```python
from build123d import *

# Parameters (mm, degrees)
SKETCH_1_W          = 20
SKETCH_1_H          = 20
EXTRUDE_1_DEPTH     = 30
SKETCH_2_R          = 5
EXTRUDE_2_DEPTH     = 50
EXTRUDE_3_DEPTH     = 20
CUT_EXTRUDE_1_REACH = 88.602
SKETCH_4_R          = 5
CUT_EXTRUDE_2_REACH = 88.348
SKETCH_5_R          = 5


with BuildPart() as part:
    # Sketch 1 → Extrude 1 (new body)
    with BuildSketch(Plane(origin=(0, 0, 0), x_dir=(1, 0, 0), z_dir=(0, 1, 0))):
        Rectangle(SKETCH_1_W, SKETCH_1_H)
    extrude(amount=EXTRUDE_1_DEPTH)

    # Sketch 2 → Extrude 2 (add)
    with BuildSketch(Plane(origin=(10, 0, 0), x_dir=(0, 0, -1), z_dir=(1, 0, 0))):
        with Locations((0, 15)):
            Circle(SKETCH_2_R)
    extrude(amount=EXTRUDE_2_DEPTH)

    # Sketch 3 → Extrude 3 (add)
    with BuildSketch(Plane(origin=(60, 0, 0), x_dir=(0, 0, -1), z_dir=(1, 0, 0))):
        Polygon((-14.14187695, 15.085535546), (0.085535546, 29.14187695), (14.14187695, 14.914464454), (-0.085535546, 0.85812305), align=None)
    extrude(amount=EXTRUDE_3_DEPTH)

    # Sketch 4 → Cut-Extrude 1 (cut, up to next)
    with BuildSketch(Plane(origin=(0, 30, 0), x_dir=(1, 0, 0), z_dir=(0, 1, 0)), mode=Mode.PRIVATE) as cut_extrude_1_sk1:
        with Locations(Location((0, 0, 0), (0, 0, 270))):
            Circle(SKETCH_4_R)
    cut_extrude_1_tool1 = extrude(cut_extrude_1_sk1.sketch, amount=-CUT_EXTRUDE_1_REACH, mode=Mode.PRIVATE) & part.part
    add(cut_extrude_1_tool1.solids().sort_by_distance((0, 30, 0))[0], mode=Mode.SUBTRACT)

    # Sketch 5 → Cut-Extrude 2 (cut, up to next)
    with BuildSketch(Plane(origin=(0, 14.704428736, 14.527621977), x_dir=(1, 0, 0), z_dir=(0, 0.7113706248059255, 0.7028170701990862)), mode=Mode.PRIVATE) as cut_extrude_2_sk1:
        with Locations(Location((70, 10.542256053, 0), (0, 0, 270))):
            Circle(SKETCH_5_R)
    cut_extrude_2_tool1 = extrude(cut_extrude_2_sk1.sketch, amount=-CUT_EXTRUDE_2_REACH, mode=Mode.PRIVATE) & part.part
    add(cut_extrude_2_tool1.solids().sort_by_distance((70, 22.113706, 7.028171))[0], mode=Mode.SUBTRACT)


solid = part.part
```
The model under review builds one solid part; all positions refer to its coordinate system, in mm. A direction names the side the tool comes from. Round coordinates to 2 decimals unless told otherwise and drop trailing zeros. Order: outer loops, then holes, each group sorted by start corner. A loop starts at its lowest first (then second) coordinate and runs counter-clockwise, first axis right, second up. Notation, with made-up numbers: M 44,73.25 L 86,73.25 A20 cw 86,78.25 Z; hole C 58,85 d3. An arc over 180 degrees is marked long. Use a Markdown table: item, result.
1) Wall thickness on line 1 along X through (y, z) = (21.25, 6.5); line 2 along X through (y, z) = (10.5, 0); line 3 along X through (y, z) = (7.75, 6): over which ranges is each line inside the solid? List them lowest first. Write a range as [from, to].
Report:
| item | result |
|---|---|
| line 1 | [-10, 10], [60, 65.01], [74.99, 80] |
| line 2 | [-10, -5], [5, 66.13], [73.87, 80] |
| line 3 | [-10, 10], [60, 80] |
2) Consider section C-C (x = 58). Write out the cut boundary in (y, z), then the cut area to 3 significant figures.
Report:
| item | result |
|---|---|
| outline | C 15,0 d10 |
| area | 78.5 mm^2 |
3) Tool access review of faces 1 (the face through (60, 15, -6)), 2 (the face through (69.86, 7.872, 7.015)), 3 (the face through (69.86, 22.128, -7.015)), 4 (the face through (0, 15, 10)): name each direction out of +Z, -Z, +X, -X, +Y, -Y from which nothing blocks a thin tool from reaching the whole face with its end or side.
Report:
| item | result |
|---|---|
| face 1 | none |
| face 2 | +Z, +X, -Y |
| face 3 | -Z, +X, +Y |
| face 4 | +Z, -X, +Y, -Y |
4) Consider section A-A (x = 0). Write out the cut boundary in (y, z), then the cut area to 3 significant figures.
Report:
| item | result |
|---|---|
| outline | M 0,-10 L 30,-10 L 30,-5 L 0,-5 Z; M 0,5 L 30,5 L 30,10 L 0,10 Z |
| area | 300 mm^2 |
5) Consider section D-D (x = 72). Write out the cut boundary in (y, z), then the cut area to 3 significant figures.
Report:
| item | result |
|---|---|
| outline | M 0.86,0.09 L 4.67,-3.77 L 18.89,10.29 L 15.09,14.14 Z; M 11.11,-10.29 L 14.91,-14.14 L 29.14,-0.09 L 25.33,3.77 Z |
| area | 217 mm^2 |
6) Insertion check: pin 1 (10 mm diameter, centred on x = 42, y = 15, fed in from +Z); pin 2 (10 mm diameter, centred on x = 3, y = 7.5, fed in from +Z); pin 3 (1 mm diameter, centred on x = 52, y = 15, fed in from -Z); pin 4 (6 mm diameter, centred on x = 41.5, z = 10, fed in from -Y). Each pin has a flat end and moves straight along its axis. Give the tip position at first contact, or say it passes through.
Report:
| item | result |
|---|---|
| pin 1 | z = 5 |
| pin 2 | z = 10 |
| pin 3 | z = -5 |
| pin 4 | through |
7) Draft analysis for pull direction Z (two halves, no side actions). For faces 5 (the face through (73.38, 17.69, -2.52)), 6 (the face through (-2, 0, -5)), 7 (the face through (34.65, 10.12, 1.08)), 8 (the face through (0, 15, -10)), state which applies: released by +Z, released by -Z, zero draft, split by the parting line, or undercut.
Report:
| item | result |
|---|---|
| face 5 | undercut |
| face 6 | zero draft |
| face 7 | split by the parting line |
| face 8 | released by -Z |
8) Consider section B-B (y = 27.5). Write out the cut boundary in (x, z), then the cut area to 3 significant figures.
Report:
| item | result |
|---|---|
| outline | M -10,-10 L 10,-10 L 10,10 L -10,10 Z; M 60,-1.71 L 80,-1.71 L 80,1.58 L 60,1.58 Z; hole C 0,0 d10 |
| area | 387 mm^2 |
